Geometry check sheet. Reference: the model listing, model coordinates, mm. A direction names the side the tool comes from. Round coordinates to 2 decimals unless told otherwise and drop trailing zeros. Write each loop counter-clockwise with the first axis right and the second up, starting at its lowest first coordinate (ties: lowest second). Pieces come first, ordered by that corner, then holes. Notation, with made-up numbers: M 81.5,51.25 L 90.5,51.25 A26 cw 90.5,74.25 Z; hole C 10,81 d8. An arc over 180 degrees is marked long. One line per item, written item: value. Start each with the question number.
1. Depth check by flat-ended pin: P1, Ø1.7, axis at x = -2, z = -4, coming from the -Y side. Enter the tip coordinate at first touch or a pass-through.
2. Access from +Z, -Z, +X, -X, +Y, -Y to the whole of each face (thin tool, end or side, straight path). Record for faces 4 (the flat face through (7.5, -5, -3)), 5 (the flat face through (0, 1, -5.7)), 6 (the cylindrical face through (9.29, -2.94, -2.81)).
3. Section check C-C (x = 9). Record the boundary of the cut face in (y, z), and give its area (3 significant figures).
4. Section check B-B (y = -2.91). Record the boundary of the cut face in (x, z).
5. Section check A-A (z = -2.8). Record the boundary of the cut face in (x, y).
6. Scan lines: probe 1 along X at (y, z) = (-5, -3.85); probe 2 along X at (y, z) = (-1.75, -3.05); probe 3 along Y at (x, z) = (-7, -1.15). Record each from-to range of solid material in increasing order. Write a range as [from, to].
7. Release check for a two-part mould opening along Y. For faces 1 (the flat face through (0, 1, 0)), 2 (the flat face through (11, -5.8, -3)), 3 (the cylindrical face through (-9.29, -2.88, -2.81)) record: pulls with the +Y half, pulls with the -Y half, needs draft (parallel to the pull), parting line crosses it, or undercut.
8. Section check D-D (x = 0). Record the boundary of the cut face in (y, z).
from build123d import *

# Parameters (mm, degrees)
BOSS_EXTRUDE1_DEPTH = 5.7
FILLET1_R           = 0.5


with BuildPart() as part:
    # Sketch1 → Boss-Extrude1 (new body)
    with BuildSketch(Plane.XY):
        with BuildLine():
            Line((7.5, -1.579841739), (7.5, 0.2))
            Line((7.5, 0.2), (-7.5, 0.2))
            Line((-7.5, 0.2), (-7.5, -1.579841739))
            ThreePointArc((-7.5, -1.579841739), (-9.289, -2.91), (-7.5, -4.240158261))
            Line((-7.5, -4.240158261), (-7.5, -5.8))
            Line((-7.5, -5.8), (-15.1, -5.8))
            Line((-15.1, -5.8), (-15.6, -5.3))
            Line((-15.6, -5.3), (-15.6, 5.3))
            Line((-15.6, 5.3), (-15.1, 5.8))
            Line((-15.1, 5.8), (15.1, 5.8))
            Line((15.1, 5.8), (15.6, 5.3))
            Line((15.6, 5.3), (15.6, -5.3))
            Line((15.6, -5.3), (15.1, -5.8))
            Line((15.1, -5.8), (7.5, -5.8))
            Line((7.5, -5.8), (7.5, -4.240158261))
            ThreePointArc((7.5, -4.240158261), (9.289, -2.91), (7.5, -1.579841739))
        make_face()
    extrude(amount=-BOSS_EXTRUDE1_DEPTH)

    # Fillet1
    fillet1_edges = [part.edges().sort_by_distance(p)[0] for p in [
        (-7.5, -1.579841739, -2.85),
        (-7.5, -4.240158261, -2.85),
        (7.5, -4.240158261, -2.85),
        (7.5, -1.579841739, -2.85),
    ]]
    fillet(fillet1_edges, radius=FILLET1_R)


solid = part.part
Result sheet:
1. P1: stops at y = 0.2
2. face 4: +Z, -Z, -Y
2. face 5: -Z, +X, -X, +Y, -Y
2. face 6: +Z, -Z
3. outline: M -5.8,-5.7 L -3.76,-5.7 L -3.76,0 L -5.8,0 Z; M -2.06,-5.7 L 5.8,-5.7 L 5.8,0 L -2.06,0 Z
3. area: 56.5 mm2
4. outline: M -15.6,-5.7 L -9.29,-5.7 L -9.29,0 L -15.6,0 Z; M 9.29,-5.7 L 15.6,-5.7 L 15.6,0 L 9.29,0 Z
5. outline: M -15.6,-5.3 L -15.1,-5.8 L -7.5,-5.8 L -7.5,-4.8 A0.5 ccw -7.97,-4.3 A1.39 cw -7.97,-1.52 A0.5 ccw -7.5,-1.02 L -7.5,0.2 L 7.5,0.2 L 7.5,-1.02 A0.5 ccw 7.97,-1.52 A1.39 cw 7.97,-4.3 A0.5 ccw 7.5,-4.8 L 7.5,-5.8 L 15.1,-5.8 L 15.6,-5.3 L 15.6,5.3 L 15.1,5.8 L -15.1,5.8 L -15.6,5.3 Z
6. probe 1: x = [-15.6, -7.5], [7.5, 15.6]
6. probe 2: x = [-15.6, -8.66], [8.66, 15.6]
6. probe 3: y = [0.2, 5.8]
7. face 1: needs draft
7. face 2: pulls with the -Y half
7. face 3: undercut
8. outline: M 0.2,-5.7 L 5.8,-5.7 L 5.8,0 L 0.2,0 Z
